Check sheet for the modelled part. Datum: model origin and axes. Units: mm. A direction names the side the tool comes from. Give positions to 0.01 mm unless a question says otherwise; leave off trailing zeros. Write each loop counter-clockwise with the first axis right and the second up, starting at its lowest first coordinate (ties: lowest second). Pieces come first, ordered by that corner, then holes. Notation, with made-up numbers: (35, 26) -> (56, 26) arc R15 ccw to (56, 44) -> close; hole circle Ø4 at (-4.75, 81). An arc over 180 degrees is marked (long way). Answer as a JSON object with one key per item and string values.
from build123d import *

# Parameters (mm, degrees)
F1_W     = 14
F1_H     = 65
F1_W_2   = 12
F1_H_2   = 23
F2_DEPTH = 1
F4_DEPTH = 10


with BuildPart() as f2:
    # F1 (on Top) → F2 (new body)
    with BuildSketch(Plane.XY):
        with Locations((7, -32.5)):
            Rectangle(F1_W, F1_H)
        with Locations((7, -17.5)):
            Rectangle(F1_W_2, F1_H_2, mode=Mode.SUBTRACT)
    extrude(amount=F2_DEPTH)

    # F3 (on face) → F4 (join)
    with BuildSketch(Plane.XY.offset(1)):
        Polygon((0, 0), (0, -65), (1, -65), (1, -29), (1, -6), (1, -1), (13, -1), (13, -6), (13, -29), (13, -65), (14, -65), (14, 0), align=None)
    extrude(amount=F4_DEPTH)


solid = f2.part
1. Sectioned sample at A-A, the plane x = 9.5. Enter the section's corners in (y, z), plus the area to 3 significant figures.
Determined:
{"outline": "(-65, 0) -> (-29, 0) -> (-29, 1) -> (-65, 1) -> close; (-6, 0) -> (0, 0) -> (0, 11) -> (-1, 11) -> (-1, 1) -> (-6, 1) -> close", "area": "52.0 mm^2"}
2. Mould release check, pull along X, two halves, no side actions. Record for faces 1 (the face through (13, -33, 5)), 2 (the face through (7, -65, 0.6)), 3 (the face through (14, -33, 5)): released by +X, released by -X, zero draft, split by the parting line, or undercut.
Determined:
{"face 1": "undercut", "face 2": "zero draft", "face 3": "released by +X"}
3. Sectioned sample at C-C, the plane y = -37.5. Enter the section's corners in (x, z), plus the area to 3 significant figures.
Determined:
{"outline": "(0, 0) -> (14, 0) -> (14, 11) -> (13, 11) -> (13, 1) -> (1, 1) -> (1, 11) -> (0, 11) -> close", "area": "34.0 mm^2"}
4. Scan lines: L1, parallel to X at y = -12, z = 2.5; L2, parallel to Y at x = 6.5, z = 2.25; L3, parallel to Z at x = 10.5, y = -59. Record each from-to range of solid material in increasing order. Write a range as [from, to].
Determined:
{"L1": "[0, 1], [13, 14]", "L2": "[-1, 0]", "L3": "[0, 1]"}
5. Sectioned sample at D-D, the plane z = 6.75. Enter the section's corners in (x, y), plus the area to 3 significant figures.
Determined:
{"outline": "(0, -65) -> (1, -65) -> (1, -1) -> (13, -1) -> (13, -65) -> (14, -65) -> (14, 0) -> (0, 0) -> close", "area": "142 mm^2"}
6. Access from +Z, -Z, +X, -X, +Y, -Y to the whole of each face (thin tool, end or side, straight path). Record for faces 4 (the face through (7, -39, 0)), 5 (the face through (7, -1, 6)).
Determined:
{"face 4": "-Z, +X, -X, +Y, -Y", "face 5": "+Z, -Y"}
7. Go/stop test with flat-tipped pins: P1, Ø3, axis at x = 11, z = 5, coming from the -Y side; P2, Ø4, axis at x = 6, y = -3.5, coming from the +Z side. Record where each tip stops, or that it passes through.
Determined:
{"P1": "y = -1", "P2": "z = 1"}
8. Sectioned sample at B-B, the plane y = -20. Enter the section's corners in (x, z).
Determined:
{"outline": "(0, 0) -> (1, 0) -> (1, 11) -> (0, 11) -> close; (13, 0) -> (14, 0) -> (14, 11) -> (13, 11) -> close"}
